from build123d import *

# Parameters (mm, degrees)
F0_W     = 88.9
F0_H     = 53.34
F1_DEPTH = 12.7
F2_W     = 78.74
F2_H     = 6.35
F3_DEPTH = 50.8
F4_W     = 63.5
F4_H     = 17.78
F5_DEPTH = 53.341
F6_W     = 2.54
F6_H     = 53.34
F7_DEPTH = 25.4
F8_SIZE  = 25.4


with BuildPart() as f1:
    # F0 (on Top) → F1 (new body)
    with BuildSketch(Plane.XY):
        Rectangle(F0_W, F0_H)
    extrude(amount=F1_DEPTH)

    # F2 (on face) → F3 (cut)
    with BuildSketch(Plane.XZ.offset(26.67)):
        with Locations((0, 5.715)):
            Rectangle(F2_W, F2_H)
    extrude(amount=-F3_DEPTH, mode=Mode.SUBTRACT)

    # F4 (on face) → F5 (cut, through all)
    with BuildSketch(Plane.XZ.offset(26.67)):
        Rectangle(F4_W, F4_H)
    extrude(amount=-F5_DEPTH, mode=Mode.SUBTRACT)

    # F6 (on face) → F7 (join)
    with BuildSketch(Plane.XY.offset(12.7)):
        Rectangle(F6_W, F6_H)
    extrude(amount=F7_DEPTH)

    # F8
    f8_edges = [f1.edges().sort_by_distance(p)[0] for p in [
        (0, -26.67, 38.1),
    ]]
    chamfer(f8_edges, length=F8_SIZE)


solid = f1.part
Could you check a few things on this model? Use its own coordinates, in mm. A direction names the side the tool comes from. Coordinates: 2 decimals unless noted, no trailing zeros. Loops run counter-clockwise (first coordinate to the right, second up) from the corner with the lowest first, then second, coordinate; pieces in that order, holes last.
1. For faces 1 (the face through (44.45, 0, 6)), 2 (the face through (23, 0, 12.7)), 3 (the face through (-1.27, 6, 25)), 4 (the face through (36, -2, 2.54)), 5 (the face through (-31.75, 2, 2)), which set-ups out of +Z, -Z, +X, -X, +Y, -Y let a thin tool reach every point of the face, with its end or its side?
2. For P1, Ø5, axis at x = 21.5, y = -19.5, coming from the -Z side; P2, Ø12, axis at y = 7, z = 23, coming from the +X side; P3, Ø8, axis at y = -4, z = 26.5, coming from the -X side, each with a flat end and sliding along its axis, tell me the tip position at first contact or that it passes through.
3. We'd pull the mould along Z, two halves only. Please class faces 6 (the face through (1.27, 6, 25)), 7 (the face through (-39.37, -2, 6)), 8 (the face through (0, 13, 38.1)): released by +Z, released by -Z, zero draft, split by the parting line, or undercut.
4. Imagine slicing it at C-C (x = 25). Please give me the cut outline in (y, z), and give its area (3 significant figures).
5. Imagine slicing it at A-A (y = -12). Please give me the cut outline in (x, z), and give its area (3 significant figures).
6. Imagine slicing it at D-D (y = 21.5). Please give me the cut outline in (x, z), and give its area (3 significant figures).
7. I need wall thicknesses on L1, parallel to X at y = 5, z = 3.5; L2, parallel to Z at x = 36, y = -2.5; L3, parallel to Z at x = -3.5, y = 7. Which ranges of each line are inside material? Lowest first, please.
8. Imagine slicing it at B-B (z = 27.5). Please give me the cut outline in (x, y).
Computed values:
1. face 1: +Z, -Z, +X, +Y, -Y
1. face 2: +Z, +X, +Y, -Y
1. face 3: +Z, -X, +Y, -Y
1. face 4: -Y
1. face 5: -Z, +Y, -Y
2. P1: stops at z = 8.89
2. P2: stops at x = 1.27
2. P3: stops at x = -1.27
3. face 6: zero draft
3. face 7: undercut
3. face 8: released by +Z
4. outline: (-26.67, 8.89) - (26.67, 8.89) - (26.67, 12.7) - (-26.67, 12.7) - close
4. area: 203 mm2
5. outline: (-44.45, 0) - (-31.75, 0) - (-31.75, 2.54) - (-39.37, 2.54) - (-39.37, 8.89) - (39.37, 8.89) - (39.37, 2.54) - (31.75, 2.54) - (31.75, 0) - (44.45, 0) - (44.45, 12.7) - (1.27, 12.7) - (1.27, 27.37) - (-1.27, 27.37) - (-1.27, 12.7) - (-44.45, 12.7) - close
5. area: 505 mm2
6. outline: (-44.45, 0) - (-31.75, 0) - (-31.75, 2.54) - (-39.37, 2.54) - (-39.37, 8.89) - (39.37, 8.89) - (39.37, 2.54) - (31.75, 2.54) - (31.75, 0) - (44.45, 0) - (44.45, 12.7) - (1.27, 12.7) - (1.27, 38.1) - (-1.27, 38.1) - (-1.27, 12.7) - (-44.45, 12.7) - close
6. area: 532 mm2
7. L1: x = -44.45 to -39.37, 39.37 to 44.45
7. L2: z = 0 to 2.54, 8.89 to 12.7
7. L3: z = 8.89 to 12.7
8. outline: (-1.27, -11.87) - (1.27, -11.87) - (1.27, 26.67) - (-1.27, 26.67) - close
